Part print with two shaded views. Sizes in mm from the minimum x, y, z corner. Give positions to 0.01 mm unless a question says otherwise; leave off trailing zeros. Loops run counter-clockwise (first coordinate to the right, second up) from the corner with the lowest first, then second, coordinate; pieces in that order, holes last. Notation, with made-up numbers: M 49.5,63.25 L 82.5,63.25 A12 ccw 82.5,76.25 Z; hole C 52,38 d11. An arc over 180 degrees is marked long. Answer as a JSON object with one key per item and string values. Group by question number.
1. Mould opens along Z. For the marked faces 1, 2 and 3 say: released by +Z, released by -Z, zero draft, split by the parting line, or undercut.
2. Drop a flat-ended pin along its axis: pin 1 Ø5 at (x, z) = (68.64, 50.8) entering from +Y. Give the stop position or say it passes through.
3. Slice it at B-B (x = 50.8). List the corners of the cut face in (y, z), then the cut area to 3 significant figures.
4. Drill centre lines: line 1 along X through (y, z) = (4.25, 50.8); line 2 along X through (y, z) = (11, 49.5) (1 decimal); line 3 along Z through (x, y) = (50.5, 10.5). Where is each one in solid material? Low to high. Write a range as [from, to].
5. Slice it at A-A (z = 50.8). List the corners of the cut face in (x, y).
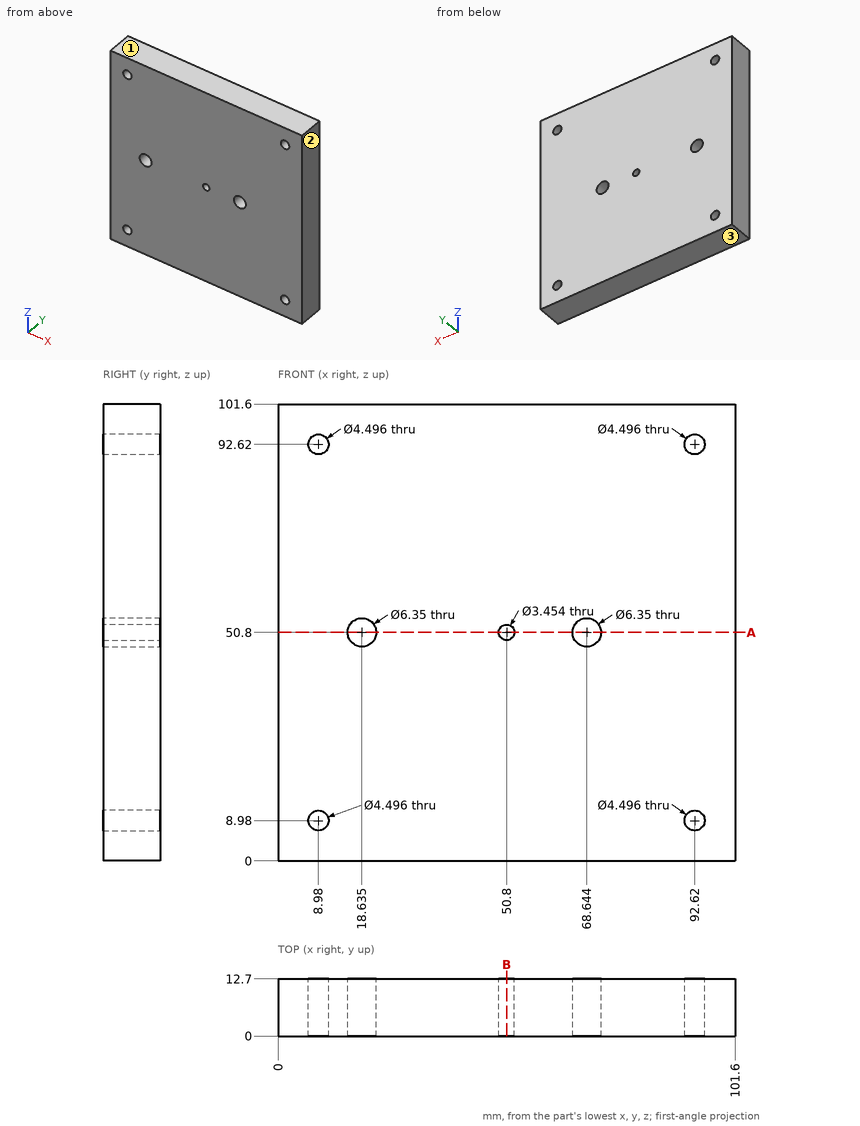
Established:
{
 "1": {"face 1": "released by +Z", "face 2": "zero draft", "face 3": "released by -Z"},
 "2": {"pin 1": "passes through"},
 "3": {"outline": "M 0,0 L 12.7,0 L 12.7,49.07 L 0,49.07 Z; M 0,52.53 L 12.7,52.53 L 12.7,101.6 L 0,101.6 Z", "area": "1,250 mm^2"},
 "4": {"line 1": "x = [0, 15.46], [21.81, 49.07], [52.53, 65.47], [71.82, 101.6]", "line 2": "x = [0, 15.7], [21.5, 49.7], [51.9, 65.7], [71.5, 101.6]", "line 3": "z = [0, 49.1], [52.5, 101.6]"},
 "5": {"outline": "M 0,0 L 15.46,0 L 15.46,12.7 L 0,12.7 Z; M 21.81,0 L 49.07,0 L 49.07,12.7 L 21.81,12.7 Z; M 52.53,0 L 65.47,0 L 65.47,12.7 L 52.53,12.7 Z; M 71.82,0 L 101.6,0 L 101.6,12.7 L 71.82,12.7 Z"}
}
